from build123d import *

# Parameters (mm, degrees)
F0_W      = 70.085093379
F0_H      = 61.8397891521
F1_DEPTH  = 54.864
F3_DEPTH  = 61.8407891521
F4_W      = 5.2283558833
F4_H      = 61.8397891521
F5_DEPTH  = 8.382
F6_W      = 5.2283558833
F6_H      = 61.8397891521
F6_W_2    = 16.4358220583
F7_DEPTH  = 38.1
F9_DEPTH  = 25.4
F10_DEPTH = 36.4407891521
F12_DEPTH = 51.054


# Not quite as in the source:
# - after a boolean that leaves OpenCascade's solid faulty, fix() repairs it


with BuildPart() as f1:
    # F0 (on Top) → F1 (new body)
    with BuildSketch(Plane.XY):
        with Locations((-35.0425466895, 30.9198945761)):
            Rectangle(F0_W, F0_H)
    extrude(amount=-F1_DEPTH)

    # F2 (on face) → F3 (cut, through all)
    with BuildSketch(Plane(origin=(0, 61.8397891521, 0), x_dir=(-1, 0, 0), z_dir=(0, 1, 0))):
        with BuildLine():
            Line((0, -54.864), (51.500908674, -54.864))
            Line((51.500908674, -54.864), (61.7086454928, -12.9319506824))
            ThreePointArc((61.7086454928, -12.9319506824), (60.5318177305, -7.5066651196), (55.5388283037, -5.08))
            Line((55.5388283037, -5.08), (52.6744276285, -5.08))
            Line((52.6744276285, -5.08), (0, -5.08))
            Line((0, -5.08), (0, -54.864))
        make_face()
        with BuildLine():
            ThreePointArc((62.0038350038, 0), (66.9968244307, -2.4266651196), (68.173652193, -7.8519506824))
            Line((68.173652193, -7.8519506824), (56.7292645574, -54.864))
            Line((56.7292645574, -54.864), (70.085093379, -54.864))
            Line((70.085093379, -54.864), (70.085093379, 0))
            Line((70.085093379, 0), (62.0038350038, 0))
        make_face()
    extrude(amount=-F3_DEPTH, mode=Mode.SUBTRACT)

    # F4 (on face) → F5 (join)
    with BuildSketch(Plane(origin=(0, 0, -54.864), x_dir=(1, 0, 0), z_dir=(0, 0, -1))):
        with Locations((-54.1150866157, -30.9198945761)):
            Rectangle(F4_W, F4_H)
    extrude(amount=F5_DEPTH)

    # F6 (on face) → F7 (join)
    with BuildSketch(Plane(origin=(0, 0, -63.246), x_dir=(1, 0, 0), z_dir=(0, 0, -1))):
        with Locations((-54.1150866157, -30.9198945761)):
            Rectangle(F6_W, F6_H)
        with Locations((-43.2829976449, -30.9198945761)):
            Rectangle(F6_W_2, F6_H)
        with Locations((-64.9471755865, -30.9198945761)):
            Rectangle(F6_W_2, F6_H)
    extrude(amount=F7_DEPTH)

    # F8 (on face) → F9 (cut)
    with BuildSketch(Plane.XZ):
        with BuildLine():
            ThreePointArc((-51.500908674, -63.4262206243), (-39.7501537967, -69.7839575966), (-35.0650866157, -82.296))
            Line((-35.0650866157, -82.296), (-35.0650866157, -63.246))
            Line((-35.0650866157, -63.246), (-51.500908674, -63.246))
            Line((-51.500908674, -63.246), (-51.500908674, -63.4262206243))
        make_face()
        with BuildLine():
            ThreePointArc((-73.1650866157, -82.296), (-68.4800194347, -69.7839575966), (-56.7292645574, -63.4262206243))
            Line((-56.7292645574, -63.4262206243), (-56.7292645574, -63.246))
            Line((-56.7292645574, -63.246), (-73.1650866157, -63.246))
            Line((-73.1650866157, -63.246), (-73.1650866157, -82.296))
        make_face()
        with BuildLine():
            Line((-35.0650866157, -101.346), (-35.0650866157, -82.296))
            ThreePointArc((-35.0650866157, -82.296), (-40.6447024341, -95.7663841816), (-54.1150866157, -101.346))
            Line((-54.1150866157, -101.346), (-35.0650866157, -101.346))
        make_face()
        with BuildLine():
            Line((-73.1650866157, -101.346), (-54.1150866157, -101.346))
            ThreePointArc((-54.1150866157, -101.346), (-67.5854707973, -95.7663841816), (-73.1650866157, -82.296))
            Line((-73.1650866157, -82.296), (-73.1650866157, -101.346))
        make_face()
    extrude(amount=-F9_DEPTH, mode=Mode.SUBTRACT)

    # F10 (cut, through all): faces of the model
    f10_faces = [f1.faces().sort_by_distance(p)[0] for p in [
        (-39.2943641898, 25.4, -67.5096317249),
        (-39.3202458526, 25.4, -97.0908407631),
        (-68.9099273788, 25.4, -97.0908407631),
        (-68.9358090416, 25.4, -67.5096317249),
    ]]
    extrude(f10_faces, amount=-F10_DEPTH, mode=Mode.SUBTRACT)

    # F11 (on face) → F12 (join)
    with BuildSketch(Plane.XZ):
        with BuildLine():
            ThreePointArc((-73.1650866157, -82.296), (-54.1150866157, -101.346), (-35.0650866157, -82.296))
            ThreePointArc((-35.0650866157, -82.296), (-39.7501537967, -69.7839575966), (-51.500908674, -63.4262206243))
            ThreePointArc((-51.500908674, -63.4262206243), (-54.1150866157, -63.246), (-56.7292645574, -63.4262206243))
            ThreePointArc((-56.7292645574, -63.4262206243), (-68.4800194347, -69.7839575966), (-73.1650866157, -82.296))
        make_face()
    extrude(amount=F12_DEPTH)

    add(f1.part.fix(), mode=Mode.REPLACE)


solid = f1.part
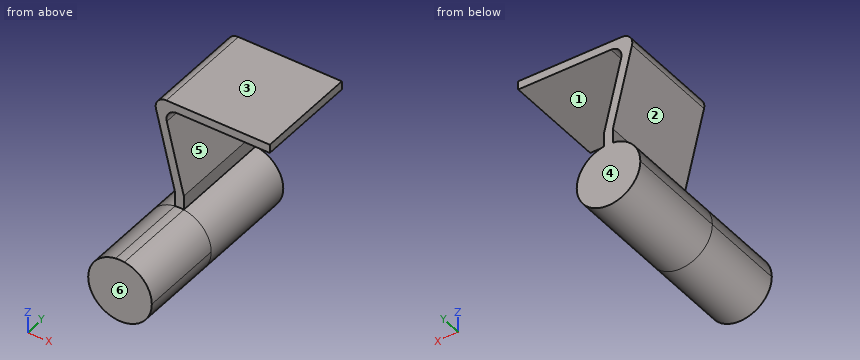
Read the model definition and answer for the solid it produces. Units are mm, in the model's axes. Face numbers are marked on the shaded views. A direction names the side the tool comes from. Round coordinates to 2 decimals unless told otherwise and drop trailing zeros. Order: outer loops, then holes, each group sorted by start corner. A loop starts at its lowest first (then second) coordinate and runs counter-clockwise, first axis right, second up.
1) For the marked faces 5 and 6, determine the directions among +Z, -Z, +X, -X, +Y, -Y from which every point of the face is accessible in a straight line to the end or side of a thin tool.
2) The part is cut by section B-B on y = -42. Write down the section's boundary in (x, z).
3) The part is cut by section A-A on x = -15. Write down the section's boundary in (y, z), plus the area to 3 significant figures.
4) Flat-ended cylindrical pins translate along their axes: pin 1 (4 mm diameter, centred on x = -10.5, y = 7.5, fed in from -Z); pin 2 (12 mm diameter, centred on x = -49.5, z = -39.5, fed in from -Y). Find the tip coordinate at first contact, or state that the pin passes through.
5) Straight lines are drawn through the part: L1, parallel to Z at x = -29.5, y = 20; L2, parallel to Y at x = -57, z = -39. For each, find the intervals that lie inside material, in ascending order.
6) The mould has two halves that part along Z. Classify the marked faces 1, 2, 3 and 4: released by +Z, released by -Z, zero draft, split by the parting line, or undercut.
Resolved:
1. face 5: +X, +Y, -Y
1. face 6: +Z, -Z, +X, -X, -Y
2. outline: circle Ø38.1 at (-54.12, -82.3)
3. outline: (0, -5.08) - (61.84, -5.08) - (61.84, 0) - (0, 0) - close
3. area: 314 mm2
4. pin 1: stops at z = -5.08
4. pin 2: stops at y = 0
5. L1: z = -5.08 to 0
5. L2: y = 0 to 61.84
6. face 1: undercut
6. face 2: undercut
6. face 3: released by +Z
6. face 4: zero draft
